Source: CAD feature listing. Evaluate the final solid. Frame: model axes, mm. A direction names the side the tool comes from. Round coordinates to 2 decimals unless told otherwise and drop trailing zeros. Write each loop counter-clockwise with the first axis right and the second up, starting at its lowest first coordinate (ties: lowest second). Pieces come first, ordered by that corner, then holes. Notation, with made-up numbers: (75, 63.25) - (126, 63.25) arc R26 cw to (126, 93.25) - close; hole circle Ø4 at (87, 7.5). An arc over 180 degrees is marked (long way). Write item = value, one per line. Start each with the question number.
Autodesk Inventor part; units mm, degrees
ref_plane "YZ Plane" through (0, 0, 0) normal (1, 0, 0) x (0, 1, 0)
ref_plane "XZ Plane" through (0, 0, 0) normal (0, 1, 0) x (-1, 0, 0)
ref_plane "XY Plane" through (0, 0, 0) normal (0, 0, 1) x (1, 0, 0)
sketch "Sketch3" plane through (0, 0, 0) normal (0, 0, 1) x (1, 0, 0)
  line L0 (-156.4592, 62.5093) -> (-106.4592, 62.5093)
  line L1 (-106.4592, 62.5093) -> (-39.3312, -17.4907)
  line L2 (-39.3312, -17.4907) -> (160.6688, -17.4907)
  line L3 (160.6688, -17.4907) -> (227.7967, 62.5093)
  line L4 (227.7967, 62.5093) -> (277.7967, 62.5093)
  point P0 (0, 0)
  dimension "d0" = 50
  dimension "d1" = 50
  dimension "d2" = 200
  dimension "d3" = 130
  dimension "d4" = 130
  dimension "d5" = 80
contour flange "Contour Flange1" sketch "Sketch3" thickness 2 bend radius 2 width 50 along (0, 0, 1) mid plane no both sides no wall seen from (-131.4592, 62.5093, 0) lies toward (0, -1, 0) curves L0 L1 L2 L3 L4
bend "Bend1"
corner "Corner1"
equation "\"d4\" = d3"
equation "\"d6\" = BendReliefWidth"
equation "\"d7\" = BendReliefDepth"
equation "\"d8\" = MinimumRemnant"
equation "\"d9\" = BendRadius"
equation "\"d11\" = BendRadius"
equation "\"d13\" = CornerReliefSize"
equation "\"d14\" = GapSize"
equation "\"d15\" = JacobiRadiusSize"
equation "\"BendRadius\" = Thickness"
equation "\"BendReliefWidth\" = Thickness"
equation "\"BendReliefDepth\" = 0.5 * Thickness"
equation "\"CornerReliefSize\" = 4 * Thickness"
equation "\"MinimumRemnant\" = 2 * Thickness"
equation "\"TransitionRadius\" = BendRadius"
equation "\"JacobiRadiusSize\" = BendRadius"
equation "\"GapSize\" = Thickness"
properties part number "handle"
(1) Ray query, L1, parallel to Y at x = -132, z = 21.5; L2, parallel to Y at x = 3, z = 42.5; L3, parallel to X at y = 39.5, z = 29. Return the intervals inside material, ascending. Write a range as from..to.
(2) Pull-direction query (X, two-part tool) for faces 1 (the flat face through (-73.053, 22.697, 24.65)), 2 (the flat face through (-74.585, 21.412, 24.65)), 3 (the flat face through (62, -18, 0)); classes: +X half, -X half, draft (parallel to the pull), parting line (faces both ways), or undercut.
(3) Section B-B (y = -6). Return the cut outline in (x, z).
(4) Section D-D (x = -58.5). Return the cut outline in (y, z), plus the area to 3 significant figures.
(5) Contact query for flat-ended pins moving along their axis: P1, Ø4, axis at y = 18.5, z = 7.5, coming from the -X side; P2, Ø3, axis at y = 34.5, z = 21, coming from the +X side; P3, Ø1.5, axis at x = 225, z = 41, coming from the +Y side. Output: stop coordinate, or through.
(6) Section A-A (z = 34). Return the cut outline in (x, y), plus the area to 3 significant figures.
(7) Reachability of faces 4 (the flat face through (62, -18, 50)), 5 (the flat face through (253, 60.509, 25)), 6 (the flat face through (253, 62.509, 25)), 7 (the flat face through (59, -17.491, 25)), 8 (the flat face through (-133, 60.509, 25)) from +Z, -Z, +X, -X, +Y, -Y: full face, straight path, thin tool, end or side. Return the list, or none.
(8) Section C-C (x = 150). Return the cut outline in (y, z).
Solution:
q1.L1 = 60.51..62.51
q1.L2 = -19.49..-17.49
q1.L3 = -89.76..-87.15, 208.49..211.1
q2.face_1 = undercut
q2.face_2 = -X half
q2.face_3 = draft
q3.outline = (-51.58, 0) - (-48.97, 0) - (-48.97, 50) - (-51.58, 50) - close; (170.31, 0) - (172.92, 0) - (172.92, 50) - (170.31, 50) - close
q4.outline = (2.24, 0) - (5.35, 0) - (5.35, 50) - (2.24, 50) - close
q4.area = 156 mm^2
q5.P1 = -73.82
q5.P2 = 208.16
q5.P3 = 60.07
q6.outline = (-156.46, 60.51) - (-108.32, 60.51) arc R2 cw to (-106.79, 59.79) - (-41.46, -18.06) arc R4 ccw to (-38.4, -19.49) - (159.74, -19.49) arc R4 ccw to (162.8, -18.06) - (228.13, 59.79) arc R2 cw to (229.66, 60.51) - (277.8, 60.51) - (277.8, 62.51) - (229.66, 62.51) arc R4 ccw to (226.6, 61.08) - (161.27, -16.78) arc R2 cw to (159.74, -17.49) - (-38.4, -17.49) arc R2 cw to (-39.93, -16.78) - (-105.26, 61.08) arc R4 ccw to (-108.32, 62.51) - (-156.46, 62.51) - close
q6.area = 1,020 mm^2
q7.face_4 = +Z, +X, -X, +Y, -Y
q7.face_5 = +Z, -Z, +X, -Y
q7.face_6 = +Z, -Z, +X, -X, +Y
q7.face_7 = +Z, -Z, +Y
q7.face_8 = +Z, -Z, -X, -Y
q8.outline = (-19.49, 0) - (-17.49, 0) - (-17.49, 50) - (-19.49, 50) - close
